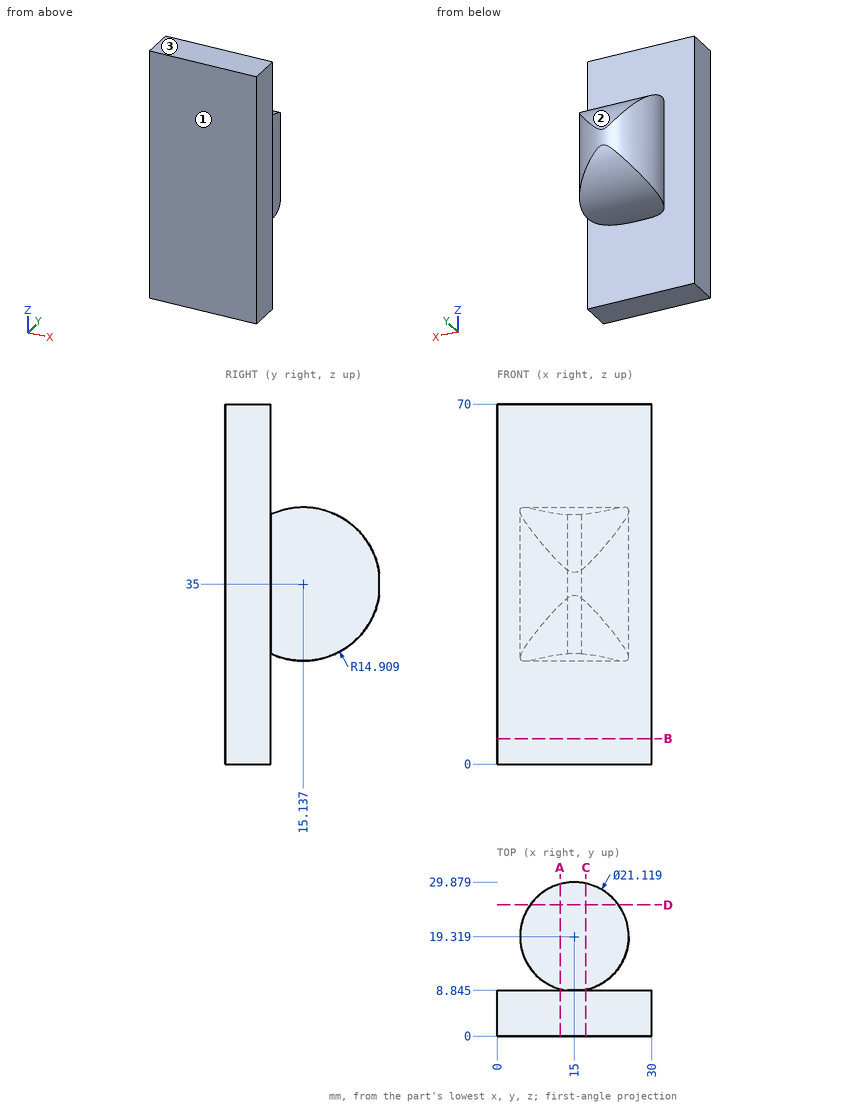
Source: three-view drawing plus pictorial views. Frame: mm from the lowest corner of the part. Give positions to 0.01 mm unless a question says otherwise; leave off trailing zeros. Order: outer loops, then holes, each group sorted by start corner. A loop starts at its lowest first (then second) coordinate and runs counter-clockwise, first axis right, second up. Notation, with made-up numbers: (37, 63.25) - (85, 63.25) arc R17 cw to (85, 90.25) - close; hole circle Ø5 at (-30, 17.25). An arc over 180 degrees is marked (long way). Put each result on its own line as item: value.
Item 1: Draft query along Y for the marked faces 1, 2 and 3. Return one class per face: +Y half, -Y half, draft (parallel to the pull), parting line (faces both ways), or undercut.
Found:
face 1: -Y half
face 2: undercut
face 3: draft
Item 2: Section query D-D, the plane y = 25.5. Return loops of the section in (x, z), then the cut area to 3 significant figures.
Found:
outline: (6.44, 24.28) - (23.56, 24.28) - (23.56, 45.72) - (6.44, 45.72) - close
area: 367 mm^2
Item 3: Ray query, L1, parallel to Y at x = 2, z = 8 (1 decimal); L2, parallel to Y at x = 12.75, z = 23.5 (1 decimal); L3, parallel to Y at x = 18, z = 40 (1 decimal). Return the intervals inside material, ascending. Write a range as from..to.
Found:
L1: y = 0..8.8
L2: y = 0..8.8, 9..24.6
L3: y = 0..8.8, 9.2..29.2
Item 4: Contact query for flat-ended pins moving along their axis: pin 1 (12 mm diameter, centred on x = 14, y = 22.5, fed in from -Z); pin 2 (12 mm diameter, centred on y = 25, z = 29, fed in from +X); pin 3 (3 mm diameter, centred on x = 19.5, y = 16.5, fed in from -Z). Output: stop coordinate, or through.
Found:
pin 1: stops at z = 20.15
pin 2: stops at x = 25.56
pin 3: stops at z = 20.09
Item 5: Section query A-A, the plane x = 12.25. Return loops of the section in (y, z) (1 decimal).
Found:
outline: (0, 0) - (8.8, 0) - (8.8, 70) - (0, 70) - close; (9.1, 21.4) arc R14.9 ccw to (29.5, 31.1) - (29.5, 38.9) arc R14.9 ccw to (9.1, 48.6) - close
Item 6: Section query C-C, the plane x = 17.25. Return loops of the section in (y, z) (1 decimal).
Found:
outline: (0, 0) - (8.8, 0) - (8.8, 70) - (0, 70) - close; (9, 21.4) arc R14.9 ccw to (29.6, 31.5) - (29.6, 38.5) arc R14.9 ccw to (9, 48.6) - close
Item 7: Section query B-B, the plane z = 5. Return loops of the section in (x, y) (1 decimal), then the cut area to 3 significant figures.
Found:
outline: (0, 0) - (30, 0) - (30, 8.8) - (0, 8.8) - close
area: 265 mm^2
